Source: CAD feature listing. Evaluate the final solid. Frame: model axes, mm. Face numbers are marked on the shaded views. A direction names the side the tool comes from. Coordinates: 2 decimals unless noted, no trailing zeros. Loops run counter-clockwise (first coordinate to the right, second up) from the corner with the lowest first, then second, coordinate; pieces in that order, holes last. Notation, with made-up numbers: (25, 84) -> (75, 84) arc R11 ccw to (75, 102) -> close; hole circle Ø11 at (2.5, 42.25). An arc over 180 degrees is marked (long way). One line per question, with ' | ' between items. Start each with the question number.
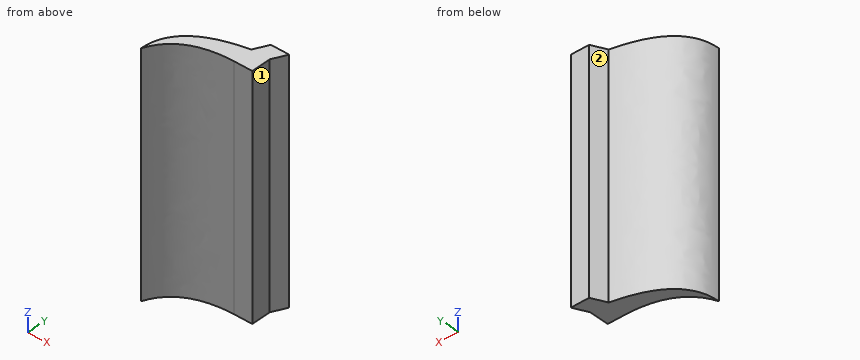
```python
from build123d import *

# Parameters (mm, degrees)
SKETCH1_W           = 58.430021541
SKETCH1_H           = 61.949414885
BOSS_EXTRUDE1_DEPTH = 750


with BuildPart() as part:
    # Sketch1 → Boss-Extrude1 (new body)
    with BuildSketch(Plane.XY):
        with BuildLine():
            add(Edge.make_bspline(
                [(-99.527538728, 54.459896253), (-100.331758171, 188.294424486), (99.44017176, 225.622803561)],
                knots=[0, 0, 0, 1, 1, 1], degree=2))
            Line((99.44017176, 225.622803561), (99.44017176, 163.673388676))
            add(Edge.make_bspline(
                [(-99.527538728, 54.459896253), (-58.241038514, 162.199954542), (99.44017176, 163.673388676)],
                knots=[0, 0, 0, 1, 1, 1], degree=2))
        make_face()
        with Locations((128.655182531, 194.648096119)):
            Rectangle(SKETCH1_W, SKETCH1_H)
        Polygon((99.44017176, 225.622803561), (121.383239857, 270.550542905), (179.813261398, 270.550542905), (157.870193301, 225.622803561), align=None)
    extrude(amount=BOSS_EXTRUDE1_DEPTH)


solid = part.part
```
(1) Ray query, L1, parallel to Y at x = 147, z = 681.5; L2, parallel to X at y = 122.5, z = 286; L3, parallel to Y at x = 44.5, z = 685.5. Return the intervals inside material, ascending.
(2) Access query for the marked faces 1 and 2. Directions: +Z, -Z, +X, -X, +Y, -Y. A direction counts if a zero-diameter tool reaches every point of the face in a straight line with its end or side. Return the directions, or none.
(3) Cut plane A-A, the plane x = 136. Return the cut outline in (y, z), and give its area (3 significant figures).
(4) Contact query for flat-ended pins moving along their axis: pin 1 Ø6 at (x, z) = (-7.5, 96.5) entering from +Y; pin 2 Ø8 at (x, z) = (-30.5, 166.5) entering from +Y; pin 3 Ø2 at (x, z) = (100.5, 261) entering from -Y. Output: stop coordinate, or through.
(5) Cut plane B-B, the plane y = 252.5. Return the cut outline in (x, z), and give its area (3 significant figures).
Here are the results:
1) L1: y = 163.67 to 270.55 | L2: x = -83.91 to -49.4 | L3: y = 159.4 to 212.4
2) face 1: +Z, -Z, +X, -Y | face 2: +Z, -Z, -X, +Y
3) outline: (163.67, 0) -> (270.55, 0) -> (270.55, 750) -> (163.67, 750) -> close | area: 80,200 mm2
4) pin 1: stops at y = 193.52 | pin 2: stops at y = 181.44 | pin 3: stops at y = 163.67
5) outline: (112.57, 0) -> (171, 0) -> (171, 750) -> (112.57, 750) -> close | area: 43,800 mm2
